Verification items for the finished model (mm, model axes). Face numbers are marked on the shaded views. A direction names the side the tool comes from. Round coordinates to 2 decimals unless told otherwise and drop trailing zeros. Write each loop counter-clockwise with the first axis right and the second up, starting at its lowest first coordinate (ties: lowest second). Pieces come first, ordered by that corner, then holes. Notation, with made-up numbers: M 47.25,-32.75 L 58.25,-32.75 A14 ccw 58.25,-27.75 Z; hole C -31.5,-33.75 d9. An arc over 180 degrees is marked long. One line per item, written item: value. Start each with the question number.
Item 1: Thickness scan on probe 1 along Z at (x, y) = (0, 8); probe 2 along Y at (x, z) = (8.75, 9.25); probe 3 along X at (y, z) = (10.5, -1). Record the ranges inside material, lowest first. Write a range as from..to.
Item 2: Gauge pin test, flat ends, axial feed: pin 1 (6 mm diameter, centred on x = -10.5, y = 7, fed in from -Z); pin 2 (2 mm diameter, centred on x = -2.5, y = 3.5, fed in from +Z); pin 3 (11 mm diameter, centred on x = 0, z = 0, fed in from -Y); pin 4 (2 mm diameter, centred on x = -6, y = 11.5, fed in from +Z). Record the tip position at first contact, or that the pin passes through.
Item 3: Section check A-A, the plane y = -2. Record the cut outline in (x, z), then the cut area to 3 significant figures.
Item 4: Tool access check on the marked faces 4 and 5. Record the directions out of +Z, -Z, +X, -X, +Y, -Y that give a thin tool (end or side, any length) a straight path to the whole face; none if there is none.
Item 5: Draft check along X on the marked faces 1, 2 and 3. Enter one of: +X half, -X half, draft (parallel to the pull), parting line (faces both ways), or undercut.
Autodesk Inventor part; units mm, degrees
ref_plane "YZ Plane" through (0, 0, 0) normal (1, 0, 0) x (0, 1, 0)
ref_plane "XZ Plane" through (0, 0, 0) normal (0, 1, 0) x (-1, 0, 0)
ref_plane "XY Plane" through (0, 0, 0) normal (0, 0, 1) x (1, 0, 0)
sketch "Skizze1" plane through (0, 0, 0) normal (0, 0, 1) x (1, 0, 0)
  line L0 (0, 146.3203) -> (0, -146.3203) construction
  line L1 (7, -16.9) -> (7, 16.9)
  line L2 (7, 16.9) -> (12.5, 16.9)
  line L3 (12.5, 16.9) -> (12.5, 15.9)
  line L4 (12.5, 15.9) -> (13.5, 15.9)
  line L5 (13.5, 15.9) -> (13.5, 14)
  line L6 (13.5, 14) -> (12.5, 14)
  line L7 (12.5, 14) -> (12.5, 13)
  line L8 (12.5, 13) -> (15, 13)
  line L9 (15, 13) -> (15, -4.65)
  line L10 (15, -4.65) -> (14.5, -5.15)
  line L11 (14.5, -5.15) -> (14.5, -5.65)
  line L12 (15, -6.4) -> (15, -6.9)
  line L13 (15, -6.9) -> (14.8, -7.1)
  line L14 (14.8, -7.1) -> (14.8, -9.7)
  line L15 (14.8, -9.7) -> (15, -9.9)
  line L16 (15, -9.9) -> (15, -10.4)
  line L17 (15, -10.4) -> (12.5, -10.4)
  line L18 (12.5, -10.4) -> (12.5, -14.7109)
  line L19 (12.5, -14.7109) -> (9.95, -15.9)
  line L20 (9.95, -15.9) -> (8.225, -15.9)
  line L21 (8.225, -15.9) -> (8.225, -16.9)
  line L22 (8.225, -16.9) -> (7, -16.9)
  line L23 (15, -6.4) -> (14.567, -5.65)
  line L24 (14.567, -5.65) -> (14.5, -5.65)
  line L25 (0, 0) -> (7, 0) construction
  dimension "d0" = 15
  dimension "d1" = 29.9
  dimension "d2" = 3.9
  dimension "d3" = 25
  dimension "d7" = 28.9
  dimension "d8" = 23.4
  dimension "d11" = 1
  dimension "d12" = 1
  dimension "d13" = 14.8
  dimension "d14" = 2.6
  dimension "d15" = 14.5
  dimension "d16" = 1.75
  dimension "d17" = 0.5
  dimension "d18" = 0.5
  dimension "d19" = 8.225
  dimension "d20" = 9.95
  dimension "d21" = 12.5
  dimension "d22" = 13.5
  dimension "d23" = 12.5
  dimension "d24" = 45
  dimension "d25" = 30
  dimension "d26" = 45
  dimension "d27" = 0.75
  dimension "d28" = 7
revolve "Umdrehung1" add sketch "Skizze1" angle 360 about axis through (0, 146.3203, 0) along (0, -1, 0)
thread "Gewinde1"
ref_plane "image plane" through (0, -32, 0) normal (0, 1, 0) x (1, 0, 0)
properties part number "ZEISS EC Epiplan-Neofluar (422320-9900-000)"
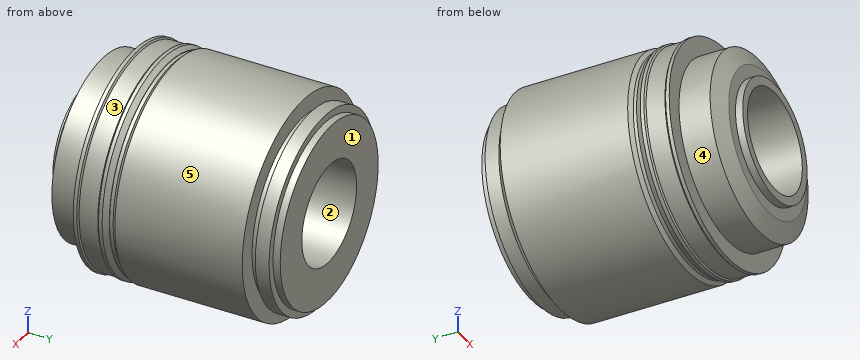
Response values:
1. probe 1: z = -15..-7, 7..15
1. probe 2: y = -10.4..13, 14..15.9
1. probe 3: x = -14.97..-6.93, 6.93..14.97
2. pin 1: stops at z = -12.99
2. pin 2: stops at z = 14.92
2. pin 3: passes through
2. pin 4: stops at z = 14.14
3. outline: C 0,0 d30; hole C 0,0 d14
3. area: 553 mm2
4. face 4: -Y
4. face 5: +Y, -Y
5. face 1: draft
5. face 2: undercut
5. face 3: parting line
